CAD build for the part. Positions are in the model's coordinates, mm. Give positions to 0.01 mm unless a question says otherwise; leave off trailing zeros. Loops run counter-clockwise (first coordinate to the right, second up) from the corner with the lowest first, then second, coordinate; pieces in that order, holes last. Notation, with made-up numbers: (34.5, 52.25) -> (45.5, 52.25) arc R24 ccw to (45.5, 71.25) -> close; hole circle Ø2 at (64, 79.25). An arc over 180 degrees is marked (long way). Use one line per item in the form item = value.
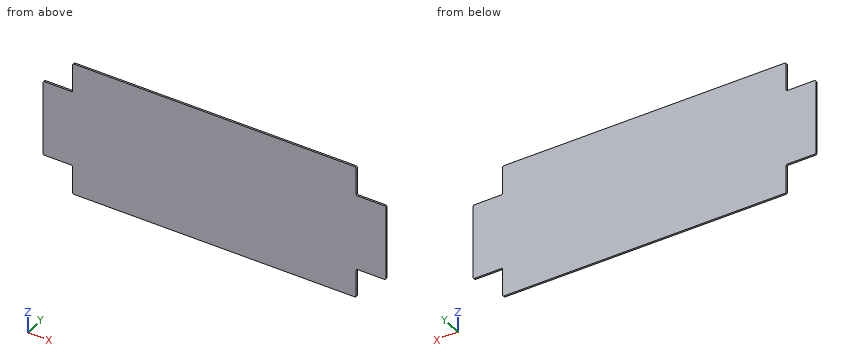
```python
from build123d import *

# Parameters (mm, degrees)
F0_W     = 1154.9995206296
F0_H     = 460.000410676
F1_DEPTH = 6
F2_W     = 100
F2_H     = 100
F3_DEPTH = 6
F4_R     = 5


with BuildPart() as f1:
    # F0 (on Front) → F1 (new body)
    with BuildSketch(Plane.XZ):
        with Locations((597.5013840944, 56.0599192977)):
            Rectangle(F0_W, F0_H)
    extrude(amount=F1_DEPTH)

    # F2 (on face) → F3 (cut)
    with BuildSketch(Plane.XZ.offset(6)):
        with Locations((70.0016237795, 236.0601246357)):
            Rectangle(F2_W, F2_H)
        with Locations((1125.0011444092, -123.9402860403)):
            Rectangle(F2_W, F2_H)
        with Locations((1125.0011444092, 236.0601246357)):
            Rectangle(F2_W, F2_H)
        with Locations((70.0016237795, -123.9402860403)):
            Rectangle(F2_W, F2_H)
    extrude(amount=-F3_DEPTH, mode=Mode.SUBTRACT)

    # F4
    f4_edges = [f1.edges().sort_by_distance(p)[0] for p in [
        (120.001624, -3, 286.060125),
        (120.001624, -3, 186.060125),
        (20.001624, -3, 186.060125),
        (20.001624, -3, -73.940286),
        (120.001624, -3, -73.940286),
        (120.001624, -3, -173.940286),
        (1075.001144, -3, -173.940286),
        (1075.001144, -3, -73.940286),
        (1175.001144, -3, -73.940286),
        (1175.001144, -3, 186.060125),
        (1075.001144, -3, 186.060125),
        (1075.001144, -3, 286.060125),
    ]]
    fillet(f4_edges, radius=F4_R)


solid = f1.part
```
1. Cut at A-A, the plane y = -3.3. Write the cut outline in (x, z), then the cut area to 3 significant figures.
Result sheet:
outline = (20, -68.94) arc R5 ccw to (25, -73.94) -> (115, -73.94) arc R5 cw to (120, -78.94) -> (120, -168.94) arc R5 ccw to (125, -173.94) -> (1070, -173.94) arc R5 ccw to (1075, -168.94) -> (1075, -78.94) arc R5 cw to (1080, -73.94) -> (1170, -73.94) arc R5 ccw to (1175, -68.94) -> (1175, 181.06) arc R5 ccw to (1170, 186.06) -> (1080, 186.06) arc R5 cw to (1075, 191.06) -> (1075, 281.06) arc R5 ccw to (1070, 286.06) -> (125, 286.06) arc R5 ccw to (120, 281.06) -> (120, 191.06) arc R5 cw to (115, 186.06) -> (25, 186.06) arc R5 ccw to (20, 181.06) -> close
area = 491,000 mm^2
2. Drop flat-ended pins along their axis: P1, Ø1.8, axis at x = 1135, y = -2.5, coming from the +Z side; P2, Ø1, axis at y = -3, z = -101.5, coming from the -X side; P3, Ø1.8, axis at x = 1145, y = -2.5, coming from the -Z side. Give the stop position or say it passes through.
Result sheet:
P1 = 186.06
P2 = 120
P3 = -73.94
3. Cut at B-B, the plane z = -103. Write the cut outline in (x, y).
Result sheet:
outline = (120, -6) -> (1075, -6) -> (1075, 0) -> (120, 0) -> close
4. Drill centre lines: line 1 (X direction, y = -2.2, z = 226); line 2 (Z direction, x = 66.5, y = -5.55); line 3 (X direction, y = -0.7, z = -76.5). Where is each one in solid material? Low to high.
Result sheet:
line_1 = 120 to 1075
line_2 = -73.94 to 186.06
line_3 = 119.37 to 1075.64
